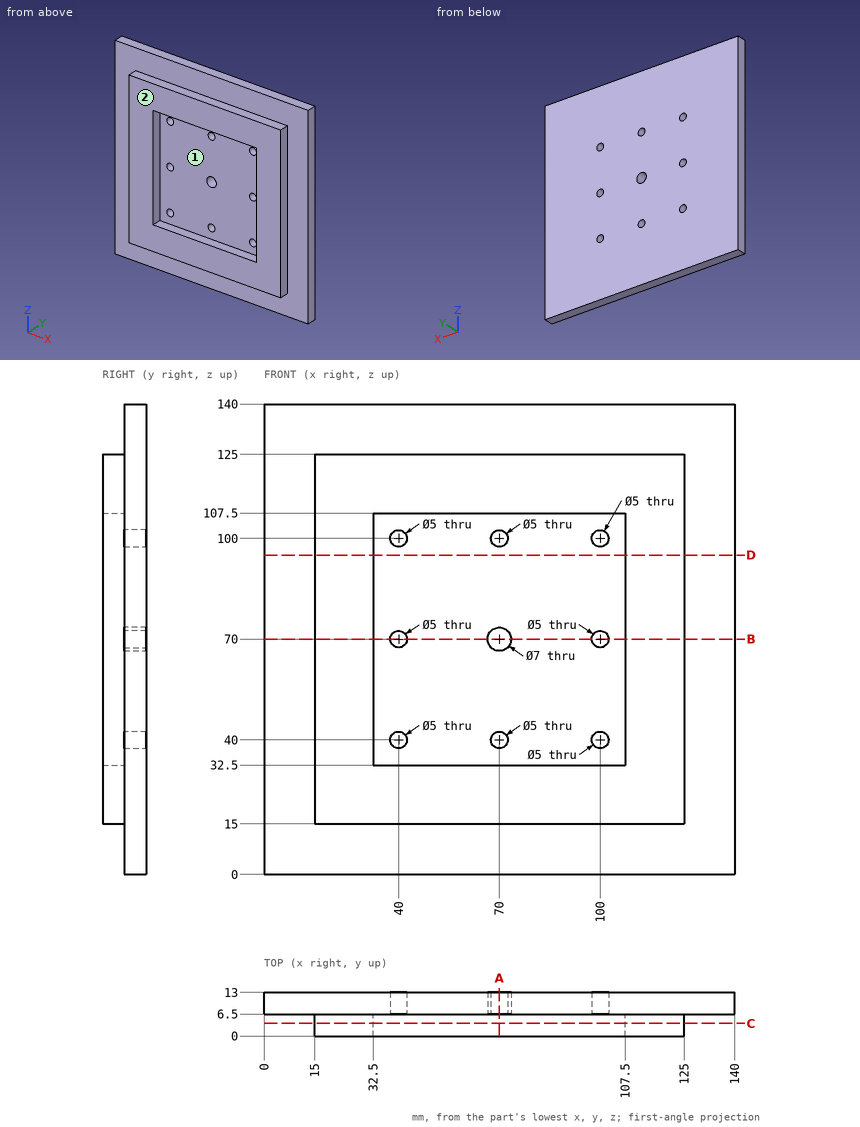
Design review of the part shown in the three views and the two pictorial views. Dimensions are in mm from the part's minimum x, y and z. A direction names the side the tool comes from. Round coordinates to 2 decimals unless told otherwise and drop trailing zeros. Write each loop counter-clockwise with the first axis right and the second up, starting at its lowest first coordinate (ties: lowest second). Pieces come first, ordered by that corner, then holes.
Item 1: For probe 1 along X at (y, z) = (9, 70); probe 2 along X at (y, z) = (9, 40), list the stretches that pass through material, from the lowest coordinate up.
Item 2: For the marked faces 1 and 2, list the 3-axis set-ups (+Z, -Z, +X, -X, +Y, -Y) from which the entire face can be reached by the end or side of a thin tool; tool diameter is ignored.
Item 3: Clearance check with flat-ended pins moving along their axes: pin 1 Ø6.5 at (x, z) = (70, 70) entering from +Y; pin 2 Ø7 at (y, z) = (2, 42.5) entering from +X; pin 3 Ø8 at (x, z) = (70, 100) entering from +Y; pin 4 Ø1.5 at (x, y) = (84.5, 2.5) entering from +Z. State where each tip first meets the part, or that it passes through.
Item 4: We need section D-D on z = 95. Write out the cut boundary in (x, y).
Item 5: We need section C-C on y = 3.75. Write out the cut boundary in (x, z).
Item 6: We need section A-A on x = 70. Write out the cut boundary in (y, z), and give its area (3 significant figures).
Item 7: We need section B-B on z = 70. Write out the cut boundary in (x, y), and give its area (3 significant figures).
Returned:
1. probe 1: x = 0 to 37.5, 42.5 to 66.5, 73.5 to 97.5, 102.5 to 140
1. probe 2: x = 0 to 37.5, 42.5 to 67.5, 72.5 to 97.5, 102.5 to 140
2. face 1: -Y
2. face 2: +Z, -Z, +X, -X, -Y
3. pin 1: passes through
3. pin 2: stops at x = 125
3. pin 3: stops at y = 13
3. pin 4: stops at z = 125
4. outline: (0, 6.5) - (15, 6.5) - (15, 0) - (32.5, 0) - (32.5, 6.5) - (107.5, 6.5) - (107.5, 0) - (125, 0) - (125, 6.5) - (140, 6.5) - (140, 13) - (0, 13) - close
5. outline: (15, 15) - (125, 15) - (125, 125) - (15, 125) - close; hole (32.5, 32.5) - (107.5, 32.5) - (107.5, 107.5) - (32.5, 107.5) - close
6. outline: (0, 15) - (6.5, 15) - (6.5, 0) - (13, 0) - (13, 37.5) - (6.5, 37.5) - (6.5, 32.5) - (0, 32.5) - close; (0, 107.5) - (6.5, 107.5) - (6.5, 102.5) - (13, 102.5) - (13, 140) - (6.5, 140) - (6.5, 125) - (0, 125) - close; (6.5, 42.5) - (13, 42.5) - (13, 66.5) - (6.5, 66.5) - close; (6.5, 73.5) - (13, 73.5) - (13, 97.5) - (6.5, 97.5) - close
6. area: 1,030 mm2
7. outline: (0, 6.5) - (15, 6.5) - (15, 0) - (32.5, 0) - (32.5, 6.5) - (37.5, 6.5) - (37.5, 13) - (0, 13) - close; (42.5, 6.5) - (66.5, 6.5) - (66.5, 13) - (42.5, 13) - close; (73.5, 6.5) - (97.5, 6.5) - (97.5, 13) - (73.5, 13) - close; (102.5, 6.5) - (107.5, 6.5) - (107.5, 0) - (125, 0) - (125, 6.5) - (140, 6.5) - (140, 13) - (102.5, 13) - close
7. area: 1,030 mm2
